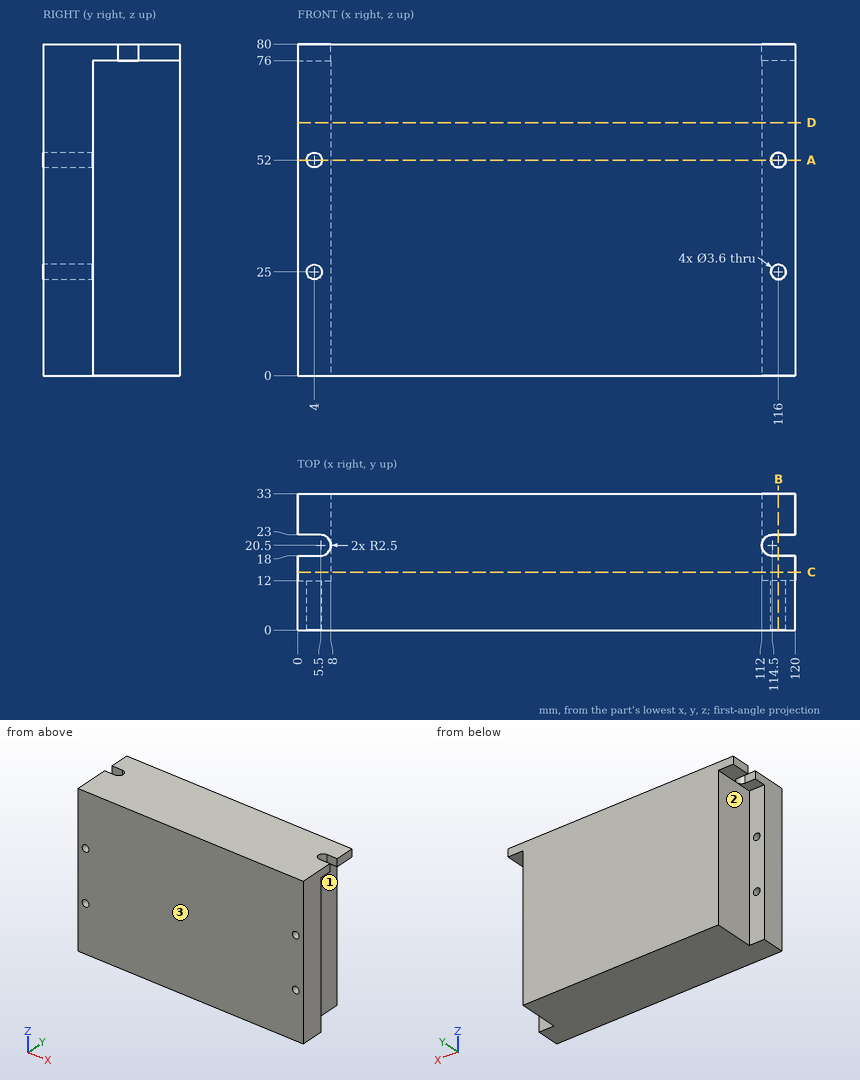
Study the drawing (mm; zero at the part's minimum x, y, z) and answer. A direction names the side the tool comes from. Coordinates: 2 decimals unless noted, no trailing zeros. Order: outer loops, then holes, each group sorted by start corner. A loop starts at its lowest first (then second) coordinate and runs counter-clockwise, first axis right, second up. Notation, with made-up numbers: (62.25, 69.25) -> (93.25, 69.25) arc R21 ccw to (93.25, 103.25) -> close; hole circle Ø2 at (-24.5, 78.5). An arc over 180 degrees is marked (long way). Answer in a Markdown table with one row per item. Add a question column.
Item 1: Which of the six approach directions +Z, -Z, +X, -X, +Y, -Y give full straight-line access (tool end or side, diameter ignored) to the marked faces 1, 2 and 3?
Item 2: Find the intervals of material crossed by L1, parallel to X at y = 6, z = 25; L2, parallel to X at y = 14, z = 39.5; L3, parallel to Y at x = 112.5, z = 58, in increasing order. Write a range as from..to.
Item 3: Find section D-D (z = 61). Write down the section's boundary in (x, y).
Item 4: Find section C-C (y = 14). Write down the section's boundary in (x, z), then the cut area to 3 significant figures.
Item 5: Find section B-B (x = 116). Write down the section's boundary in (y, z), then the cut area to 3 significant figures.
Item 6: Find section A-A (z = 52). Write down the section's boundary in (x, y), then the cut area to 3 significant figures.
Item 7: Each of these flat-tipped pins is pushed along its axis until it touches: P1, Ø8, axis at y = 27, z = 29, coming from the +X side; P2, Ø2.5, axis at x = 3.5, y = 15, coming from the -Z side; P3, Ø4.5, axis at x = 4, z = 25, coming from the +Y side. Where does it stop, or does it pass through?
Result set:
| question | item | result |
|---|---|---|
| 1 | face 1 | -Z, +X, +Y |
| 1 | face 2 | -Z, -X, +Y |
| 1 | face 3 | +Z, -Z, +X, -X, -Y |
| 2 | L1 | x = 0..2.2, 5.8..114.2, 117.8..120 |
| 2 | L2 | x = 8..112 |
| 2 | L3 | y = 0..12 |
| 3 | outline | (0, 0) -> (120, 0) -> (120, 12) -> (112, 12) -> (112, 33) -> (8, 33) -> (8, 12) -> (0, 12) -> close |
| 4 | outline | (0, 76) -> (8, 76) -> (8, 0) -> (112, 0) -> (112, 76) -> (120, 76) -> (120, 80) -> (0, 80) -> close |
| 4 | area | 8,380 mm² |
| 5 | outline | (0, 0) -> (12, 0) -> (12, 23.2) -> (0, 23.2) -> close; (0, 26.8) -> (12, 26.8) -> (12, 50.2) -> (0, 50.2) -> close; (0, 53.8) -> (12, 53.8) -> (12, 76) -> (18, 76) -> (18, 80) -> (0, 80) -> close; (23, 76) -> (33, 76) -> (33, 80) -> (23, 80) -> close |
| 5 | area | 938 mm² |
| 6 | outline | (0, 0) -> (2.2, 0) -> (2.2, 12) -> (0, 12) -> close; (5.8, 0) -> (114.2, 0) -> (114.2, 12) -> (112, 12) -> (112, 33) -> (8, 33) -> (8, 12) -> (5.8, 12) -> close; (117.8, 0) -> (120, 0) -> (120, 12) -> (117.8, 12) -> close |
| 6 | area | 3,540 mm² |
| 7 | P1 | stops at x = 112 |
| 7 | P2 | stops at z = 76 |
| 7 | P3 | stops at y = 12 |
